```python
from build123d import *

# Parameters (mm, degrees)
BOSS_EXTRUDE1_DEPTH = 5


with BuildPart() as part:
    # Sketch1 → Boss-Extrude1 (new body)
    with BuildSketch(Plane.XY):
        with BuildLine():
            Line((-24.323076923, 14.485250559), (-24.323076923, 13.317117605))
            ThreePointArc((-24.323076923, 13.317117605), (-24.377668127, 12.853022124), (-24.538461538, 12.414262174))
            ThreePointArc((-24.538461538, 12.414262174), (-26.749370949, 6.381312862), (-27.5, 0))
            Line((-27.5, 0), (-24.5, 0))
            ThreePointArc((-24.5, 0), (-23.831257754, 5.685169641), (-21.861538462, 11.059979028))
            ThreePointArc((-21.861538462, 11.059979028), (-21.459554932, 12.156878903), (-21.323076923, 13.317117605))
            Line((-21.323076923, 13.317117605), (-21.323076923, 14.485250559))
            ThreePointArc((-21.323076923, 14.485250559), (-21.059553746, 16.08705807), (-20.296762002, 17.52002022))
            ThreePointArc((-20.296762002, 17.52002022), (-10.731713115, 22.70625472), (0, 24.5))
            ThreePointArc((0, 24.5), (10.731713115, 22.70625472), (20.296762002, 17.52002022))
            ThreePointArc((20.296762002, 17.52002022), (21.059553746, 16.08705807), (21.323076923, 14.485250559))
            Line((21.323076923, 14.485250559), (21.323076923, 13.317117605))
            ThreePointArc((21.323076923, 13.317117605), (21.459554932, 12.156878903), (21.861538462, 11.059979028))
            ThreePointArc((21.861538462, 11.059979028), (23.831257754, 5.685169641), (24.5, 0))
            Line((24.5, 0), (27.5, 0))
            ThreePointArc((27.5, 0), (26.749370949, 6.381312862), (24.538461538, 12.414262174))
            ThreePointArc((24.538461538, 12.414262174), (24.377668127, 12.853022124), (24.323076923, 13.317117605))
            Line((24.323076923, 13.317117605), (24.323076923, 14.485250559))
            ThreePointArc((24.323076923, 14.485250559), (23.831147361, 17.247292972), (22.41585735, 19.669652807))
            ThreePointArc((22.41585735, 19.669652807), (11.872078566, 25.486081718), (0, 27.5))
            ThreePointArc((0, 27.5), (-11.872078566, 25.486081718), (-22.41585735, 19.669652807))
            ThreePointArc((-22.41585735, 19.669652807), (-23.831147361, 17.247292972), (-24.323076923, 14.485250559))
        make_face()
    extrude(amount=BOSS_EXTRUDE1_DEPTH)


solid = part.part
```
Can you work these out from the model? Positions are in its coordinate system, mm. A direction names the side the tool comes from. Round coordinates to 2 decimals unless told otherwise and drop trailing zeros. Loops run counter-clockwise (first coordinate to the right, second up) from the corner with the lowest first, then second, coordinate; pieces in that order, holes last.
Item 1: Suppose I cut it at C-C, the plane y = 23. Write out the boundary of the cut face in (x, z).
Item 2: Suppose I cut it at D-D, the plane x = -14.5. Write out the boundary of the cut face in (y, z).
Item 3: Will these pins go through, and if not, where does the flat tip stop? pin 1 Ø2 at (y, z) = (20, 4) entering from +X; pin 2 Ø1.5 at (x, z) = (-10.5, 4) entering from +Y; pin 3 Ø1.3 at (y, z) = (13.5, 2.5) entering from +X; pin 4 Ø2 at (x, y) = (10.5, 20) entering from -Z.
Item 4: Please list where these lines run through material, in increasing order: L1, parallel to X at y = 14.25, z = 2.8; L2, parallel to X at y = 5.5, z = 0.8; L3, parallel to Y at x = 16, z = 0.7.
Item 5: Which directions (+Z, -Z, +X, -X, +Y, -Y) give clear straight access to the entire face, cutting with the end or side of a thin tool? Please do faces 1 (the cylindrical face through (-21.067, 16.065, 2.465)), 2 (the flat face through (-2, 25, 5)), 3 (the flat face through (24.323, 14, 2)).
Item 6: If we mould it in two halves opening along X, with no side actions, what happens to faces 4 (the cylindrical face through (23.812, 5.763, 2.465)), 5 (the cylindrical face through (-21.463, 12.141, 2.465)), 6 (the flat face through (-26, 0, 2)), 7 (the flat face through (-24.323, 14, 2))? For each: +X half, -X half, draft (parallel to the pull), parting line (faces both ways), or undercut.
Item 7: Suppose I cut it at A-A, the plane z = 0.95. Write out the boundary of the cut face in (x, y), then the cut area to 3 significant figures.
Item 8: Suppose I cut it at B-B, the plane y = 7.5. Write out the boundary of the cut face in (x, z).
Reported:
1. outline: (-17.43, 0) - (-9.84, 0) - (-9.84, 5) - (-17.43, 5) - close; (9.84, 0) - (17.43, 0) - (17.43, 5) - (9.84, 5) - close
2. outline: (21.14, 0) - (24.45, 0) - (24.45, 5) - (21.14, 5) - close
3. pin 1: stops at x = 22.93
3. pin 2: stops at y = 26.15
3. pin 3: stops at x = 24.38
3. pin 4: passes through
4. L1: x = -24.32 to -21.32, 21.32 to 24.32
4. L2: x = -26.94 to -23.87, 23.87 to 26.94
4. L3: y = 20.36 to 23.75
5. face 1: +Z, -Z, -Y
5. face 2: +Z, +X, -X, +Y, -Y
5. face 3: +Z, -Z, +X, +Y
6. face 4: undercut
6. face 5: undercut
6. face 6: draft
6. face 7: -X half
7. outline: (-27.5, 0) - (-24.5, 0) arc R24.5 cw to (-21.86, 11.06) arc R5 ccw to (-21.32, 13.32) - (-21.32, 14.49) arc R5 cw to (-20.3, 17.52) arc R33 cw to (20.3, 17.52) arc R5 cw to (21.32, 14.49) - (21.32, 13.32) arc R5 ccw to (21.86, 11.06) arc R24.5 cw to (24.5, 0) - (27.5, 0) arc R27.5 ccw to (24.54, 12.41) arc R2 cw to (24.32, 13.32) - (24.32, 14.49) arc R8 ccw to (22.42, 19.67) arc R36 ccw to (-22.42, 19.67) arc R8 ccw to (-24.32, 14.49) - (-24.32, 13.32) arc R2 cw to (-24.54, 12.41) arc R27.5 ccw to start
7. area: 255 mm2
8. outline: (-26.46, 0) - (-23.32, 0) - (-23.32, 5) - (-26.46, 5) - close; (23.32, 0) - (26.46, 0) - (26.46, 5) - (23.32, 5) - close
